Could you check a few things on this model? Use its own coordinates, in mm. A direction names the side the tool comes from. Give positions to 0.01 mm unless a question says otherwise; leave off trailing zeros. Write each loop counter-clockwise with the first axis right and the second up, starting at its lowest first coordinate (ties: lowest second). Pieces come first, ordered by that corner, then holes. Notation, with made-up numbers: M -2.5,-4.75 L 40.5,-4.75 A28 cw 40.5,23.25 Z; hole C 49,28 d3. An arc over 180 degrees is marked long. One line per item, written item: value.
```python
from build123d import *

# Parameters (mm, degrees)
SCHIZZO1_W                   = 16
SCHIZZO1_H                   = 3
SCHIZZO2_R                   = 8
ESTRUSIONE_ESTRUSIONE1_DEPTH = 10
FORO_3_9_3_9_1_D             = 3.9
FORO_8_0_8_1_D               = 8
FORO_PER_VITE_M3_1_REACH     = 31.933
FORO_PER_VITE_M3_1_BORE_R    = 1.62


with BuildPart() as part:
    # Schizzo1 → Rivoluzione1 (revolve)
    with BuildSketch(Plane(origin=(0, 0, 0), x_dir=(1, 0, 0), z_dir=(0, 1, 0))):
        with Locations((8, -1.5)):
            Rectangle(SCHIZZO1_W, SCHIZZO1_H)
    revolve(axis=Axis((0, 0, 0), (0, 0, 1)))

    # Schizzo2 → Estrusione-Estrusione1 (add)
    with BuildSketch(Plane.XY.offset(3)):
        Circle(SCHIZZO2_R)
    extrude(amount=ESTRUSIONE_ESTRUSIONE1_DEPTH)

    # Foro Ø3.9 (3.9)-1 (through all)
    with Locations(Plane.XY.offset(3)):
        with Locations((12, 0), (0, 12), (-12, 0), (0, -12)):
            Hole(FORO_3_9_3_9_1_D / 2)

    # Foro Ø8.0 (8)-1 (through all)
    with Locations(Plane.XY.offset(13)):
        with Locations((0, 0)):
            Hole(FORO_8_0_8_1_D / 2)

    # Foro per Vite M3-1 bore (on position points) → Foro per Vite M3-1 (cut, up to next)
    with BuildSketch(Plane(origin=(-8, 0, 8), x_dir=(0, 0, -1), z_dir=(-1, 0, 0)), mode=Mode.PRIVATE) as foro_per_vite_m3_1_sk1:
        Circle(FORO_PER_VITE_M3_1_BORE_R)
    foro_per_vite_m3_1_tool1 = extrude(foro_per_vite_m3_1_sk1.sketch, amount=-FORO_PER_VITE_M3_1_REACH, mode=Mode.PRIVATE) & part.part
    add(foro_per_vite_m3_1_tool1.solids().sort_by_distance((-8, 0, 8))[0], mode=Mode.SUBTRACT)


solid = part.part
```
1) If we section it at A-A, the plane y = 0: Write out the boundary of the cut face in (x, z).
Outcome:
outline: M -16,0 L -13.95,0 L -13.95,3 L -16,3 Z; M -10.05,0 L -4,0 L -4,6.38 L -8,6.38 L -8,3 L -10.05,3 Z; M -8,9.62 L -4,9.62 L -4,13 L -8,13 Z; M 4,0 L 10.05,0 L 10.05,3 L 8,3 L 8,13 L 4,13 Z; M 13.95,0 L 16,0 L 16,3 L 13.95,3 Z
2) If we section it at D-D, the plane y = 13: Write out the boundary of the cut face in (x, z).
Outcome:
outline: M -9.33,0 L -1.67,0 L -1.67,3 L -9.33,3 Z; M 1.67,0 L 9.33,0 L 9.33,3 L 1.67,3 Z
3) If we section it at B-B, the plane z = 2.5: Write out the boundary of the cut face in (x, y).
Outcome:
outline: C 0,0 d32; hole C -12,0 d3.9; hole C 0,0 d8; hole C 0,-12 d3.9; hole C 0,12 d3.9; hole C 12,0 d3.9
4) On a 3-axis mill with a long thin cutter (end or side, diameter ignored), from which of +Z, -Z, +X, -X, +Y, -Y can I reach the whole of each face in a straight line? I mean faces 1 (the face through (-10.563, 1.318, 1.479)), 2 (the face through (7.3, 3.8, 3)). Say none if no direction works.
Outcome:
face 1: +Z, -Z
face 2: +Z
5) We'd pull the mould along Z, two halves only. Please class faces 3 (the face through (13.437, 1.318, 1.479)), 4 (the face through (-3, -3, 0)), 5 (the face through (-5.86, -0.07, 9.62)): pulls with the +Z half, pulls with the -Z half, needs draft (parallel to the pull), parting line crosses it, or undercut.
Outcome:
face 3: needs draft
face 4: pulls with the -Z half
face 5: undercut
6) If we section it at C-C, the plane x = -12: Write out the boundary of the cut face in (y, z), then the cut area to 3 significant figures.
Outcome:
outline: M -10.58,0 L -1.95,0 L -1.95,3 L -10.58,3 Z; M 1.95,0 L 10.58,0 L 10.58,3 L 1.95,3 Z
area: 51.8 mm^2
7) I'm going to push flat-ended pins straight in: pin 1 (4 mm diameter, centred on x = -10.5, z = 11, fed in from +Y); pin 2 (1.5 mm diameter, centred on y = 9.5, z = 3.5, fed in from -X); pin 3 (1 mm diameter, centred on x = -1.5, z = 1.5, fed in from -Y); pin 4 (5 mm diameter, centred on x = 12, y = 0, fed in from +Z). Where does each tip first touch, or does it pass through?
Outcome:
pin 1: passes through
pin 2: stops at x = -13.27
pin 3: stops at y = -15.97
pin 4: stops at z = 3
8) Please list where these lines run through material, in increasing order: L1, parallel to Z at x = -4.85, y = 0; L2, parallel to Z at x = -15, y = 3; L3, parallel to X at y = -3, z = 10. Write a range as from..to.
Outcome:
L1: z = 0..6.38, 9.62..13
L2: z = 0..3
L3: x = -7.42..-2.65, 2.65..7.42
